Work out the finished part from the listing and answer in its coordinate system (mm). A direction names the side the tool comes from. Give positions to 0.01 mm unless a question says otherwise; leave off trailing zeros. Order: outer loops, then holes, each group sorted by start corner. A loop starts at its lowest first (then second) coordinate and runs counter-clockwise, first axis right, second up. Notation, with made-up numbers: (40.5, 79.5) - (47.5, 79.5) arc R22 ccw to (47.5, 90.5) - close; hole circle Ø4 at (-3, 86). An arc over 180 degrees is marked (long way). Return JSON: item names as keys, results as strings. Group by question number.
from build123d import *

# Parameters (mm, degrees)
EXTRUDE_1_DEPTH   = 2
HOLE_WIZARD_M61_D = 6.6
CHAMFER_1_SIZE    = 2


with BuildPart() as part:
    # Эскиз1 → Бобышка-Вытянуть1 (new body)
    with BuildSketch(Plane(origin=(0, 0, 0), x_dir=(1, 0, 0), z_dir=(0, 0, -1))):
        Polygon((-30, 90), (30, 90), (30, 60), (15, 60), (15, 0), (-15, 0), (-15, 60), (-30, 60), align=None)
    extrude(amount=EXTRUDE_1_DEPTH)

    # Отверстие с зазором M61 (through all)
    with Locations(Plane(origin=(0, 0, -2), x_dir=(1, 0, 0), z_dir=(0, 0, -1))):
        with Locations((0, 15), (-15, 75), (15, 75), (0, 45)):
            Hole(HOLE_WIZARD_M61_D / 2)

    # Фаска1
    chamfer_1_edges = [part.edges().sort_by_distance(p)[0] for p in [
        (-30, -60, -1),
        (-30, -90, -1),
        (30, -90, -1),
        (30, -60, -1),
        (15, 0, -1),
        (-15, 0, -1),
    ]]
    chamfer(chamfer_1_edges, length=CHAMFER_1_SIZE)


solid = part.part
1. A tool of negligible diameter and unlimited length cuts with its end or side. For faces 5 (the flat face through (0, -90, -1)), 6 (the flat face through (-21, -60, -1)), 7 (the flat face through (15, -31, -1)), from which of +Z, -Z, +X, -X, +Y, -Y can it reach the whole face along a straight path? Write none if from no direction.
2. Determine the mould class of faces 1 (the cylindrical face through (2.43, -17.23, -0.99)), 2 (the flat face through (29, -61, -1)), 3 (the flat face through (30, -75, -1)), 4 (the cylindrical face through (0.43, -48.27, -0.99)) for opening direction Y: released by +Y, released by -Y, zero draft, split by the parting line, or undercut.
3. The part is cut by section D-D (y = -15). Give the vertices of the cut face in (x, z), and give its area (3 significant figures).
4. Consider probe 1 along X at (y, z) = (-75, -1.6); probe 2 along Y at (x, z) = (0, -1.25); probe 3 along X at (y, z) = (-45, -0.1). Determine where each line is inside the solid, lowest interval first. Write a range as from..to.
5. The part is cut by section A-A (y = -75). Give the vertices of the cut face in (x, z), and give its area (3 significant figures).
6. The part is cut by section C-C (z = -1.1). Give the vertices of the cut face in (x, y), and give its area (3 significant figures).
7. Each of these flat-tipped pins is pushed along its axis until it touches: pin 1 (1 mm diameter, centred on x = 22.5, z = -1, fed in from +Y); pin 2 (8.5 mm diameter, centred on x = 0, y = -45, fed in from +Z); pin 3 (1 mm diameter, centred on y = -26.5, z = -1, fed in from +X); pin 4 (1 mm diameter, centred on y = -23, z = -1.5, fed in from -X). Where does it stop, or does it pass through?
8. The part is cut by section B-B (x = 0). Give the vertices of the cut face in (y, z), and give its area (3 significant figures).
Answers:
{
 "1": {"face 5": "+Z, -Z, +X, -X, -Y", "face 6": "+Z, -Z, -X, +Y", "face 7": "+Z, -Z, +X, +Y"},
 "2": {"face 1": "undercut", "face 2": "released by +Y", "face 3": "zero draft", "face 4": "undercut"},
 "3": {"outline": "(-15, -2) - (-3.3, -2) - (-3.3, 0) - (-15, 0) - close; (3.3, -2) - (15, -2) - (15, 0) - (3.3, 0) - close", "area": "46.8 mm^2"},
 "4": {"probe 1": "x = -30..-18.3, -11.7..11.7, 18.3..30", "probe 2": "y = -90..-48.3, -41.7..-18.3, -11.7..0", "probe 3": "x = -15..-3.3, 3.3..15"},
 "5": {"outline": "(-30, -2) - (-18.3, -2) - (-18.3, 0) - (-30, 0) - close; (-11.7, -2) - (11.7, -2) - (11.7, 0) - (-11.7, 0) - close; (18.3, -2) - (30, -2) - (30, 0) - (18.3, 0) - close", "area": "93.6 mm^2"},
 "6": {"outline": "(-30, -88) - (-28, -90) - (28, -90) - (30, -88) - (30, -62) - (28, -60) - (15, -60) - (15, -2) - (13, 0) - (-13, 0) - (-15, -2) - (-15, -60) - (-28, -60) - (-30, -62) - close; hole circle Ø6.6 at (-15, -75); hole circle Ø6.6 at (0, -45); hole circle Ø6.6 at (0, -15); hole circle Ø6.6 at (15, -75)", "area": "3,450 mm^2"},
 "7": {"pin 1": "stops at y = -60", "pin 2": "stops at z = 0", "pin 3": "stops at x = 15", "pin 4": "stops at x = -15"},
 "8": {"outline": "(-90, -2) - (-48.3, -2) - (-48.3, 0) - (-90, 0) - close; (-41.7, -2) - (-18.3, -2) - (-18.3, 0) - (-41.7, 0) - close; (-11.7, -2) - (0, -2) - (0, 0) - (-11.7, 0) - close", "area": "154 mm^2"}
}
